The listing builds one solid part. Answer for the finished solid, in the listing's coordinates (mm). Coordinates: 2 decimals unless noted, no trailing zeros. Write each loop counter-clockwise with the first axis right and the second up, starting at its lowest first coordinate (ties: lowest second). Pieces come first, ordered by that corner, then holes.
from build123d import *

# Parameters (mm, degrees)
F0_R     = 38.1
F1_DEPTH = 101.6
F2_R     = 38.1
F3_SIZE  = 10.16


with BuildPart() as f1:
    # F0 (on Right) → F1 (new body)
    with BuildSketch(Plane.YZ):
        Circle(F0_R)
    extrude(amount=F1_DEPTH)

    # F2
    f2_edges = [f1.edges().sort_by_distance(p)[0] for p in [
        (101.6, -38.1, 0),
    ]]
    fillet(f2_edges, radius=F2_R)

    # F3
    f3_edges = [f1.edges().sort_by_distance(p)[0] for p in [
        (0, -38.1, 0),
    ]]
    chamfer(f3_edges, length=F3_SIZE)


solid = f1.part
Q1. Determine the mould class of faces 1 (the face through (36.457, -30.235, -23.183)), 2 (the face through (0, 0, 0)) for opening direction Z: released by +Z, released by -Z, zero draft, split by the parting line, or undercut.
Answers below:
face 1: split by the parting line
face 2: zero draft
Q2. Find the intervals of material crossed by probe 1 along Z at (x, y) = (78.5, -17); probe 2 along Z at (x, y) = (15, -13); probe 3 along X at (y, z) = (23.5, -25), in increasing order.
Answers below:
probe 1: z = -30.62 to 30.62
probe 2: z = -35.81 to 35.81
probe 3: x = 6.37 to 80.06
Q3. The part is cut by section A-A, the plane z = 0. Write down the section's boundary in (x, y), then the cut area to 3 significant figures.
Answers below:
outline: (0, -27.94) - (10.16, -38.1) - (63.5, -38.1) arc R38.1 ccw to (63.5, 38.1) - (10.16, 38.1) - (0, 27.94) - close
area: 7,020 mm2
Q4. Given pin 1 (3 mm diameter, centred on y = -30.5, z = 17.5, fed in from -X); pin 2 (5 mm diameter, centred on x = 57.5, z = -30, fed in from -Y); pin 3 (6 mm diameter, centred on x = 44, y = 11.5, fed in from +Z); pin 4 (2 mm diameter, centred on y = -1.5, z = -15.5, fed in from -X), each flat-ended and moving along its own axis, determine where each tip first touches the part or whether it passes through.
Answers below:
pin 1: stops at x = 5.72
pin 2: stops at y = -26.37
pin 3: stops at z = 37.14
pin 4: stops at x = 0
Q5. The part is cut by section C-C, the plane x = 61.5. Write down the section's boundary in (y, z), then the cut area to 3 significant figures.
Answers below:
outline: circle Ø76.2 at (0, 0)
area: 4,560 mm2
